The listing builds one solid part. Answer for the finished solid, in the listing's coordinates (mm). A direction names the side the tool comes from. Round coordinates to 2 decimals unless told otherwise and drop trailing zeros. Write each loop counter-clockwise with the first axis right and the second up, starting at its lowest first coordinate (ties: lowest second). Pieces come first, ordered by that corner, then holes.
(1) Each of these flat-tipped pins is pushed along its axis until it touches: pin 1 Ø2 at (x, y) = (-2.5, 9) entering from +Z; pin 2 Ø2 at (x, y) = (-8.5, 7) entering from +Z; pin 3 Ø2 at (y, z) = (11, 6) entering from -X. Where does it stop, or does it pass through?
(2) A cutting plane is placed at D-D, the plane z = -7. Give the vertices of the cut face in (x, y), and give its area (3 significant figures).
(3) Find the intervals of material crossed by probe 1 along Y at (x, z) = (0, 10); probe 2 along X at (y, z) = (9.75, 0) (3 decimals); probe 3 along X at (y, z) = (2.5, -4.75), in increasing order.
(4) The mould has two halves that part along X. Classify faces 3 (the face through (5.554, 7.148, -13.394)), 4 (the face through (8.12, 12.04, -9.35)): +X half, -X half, draft (parallel to the pull), parting line (faces both ways), or undercut.
(5) A cutting plane is placed at A-A, the plane x = 5.5. Give the vertices of the cut face in (y, z), and give its area (3 significant figures).
(6) For faces 1 (the face through (0, 1, 2.502)), 2 (the face through (4.8, 9.5, -4.6)), determine the directions among +Z, -Z, +X, -X, +Y, -Y from which every point of the face is accessible in a straight line to the end or side of a thin tool.
(7) A cutting plane is placed at B-B, the plane z = 0. Give the vertices of the cut face in (x, y) (3 decimals), and give its area (3 significant figures).
(8) A cutting plane is placed at C-C, the plane y = 11. Give the number of separate pieces and of enclosed holes in the cut face, and give its area (3 significant figures).
from build123d import *
from build123d.topology import SkipClean

# Parameters (mm, degrees)
CROQUIS1_R              = 14.5
SALIENTE_EXTRUIR1_DEPTH = 14.5
CORTAR_EXTRUIR1_DEPTH   = 26.11473671
CORTAR_EXTRUIR2_DEPTH   = 26.11473671
CORTAR_EXTRUIR3_DEPTH   = 5
MATRIZL1_COUNT          = 2
MATRIZL1_PITCH          = 12.728
MATRIZL1_COUNT_DIR2     = 2
MATRIZL1_PITCH_DIR2     = 12.728
CROQUIS6_R              = 2
CORTAR_EXTRUIR4_DEPTH   = 11.998295581
CORTAR_EXTRUIR5_DEPTH   = 1
CORTAR_EXTRUIR9_DEPTH   = 1.9


with BuildPart() as part:
    # Croquis1 → Saliente-Extruir1 (new body)
    with BuildSketch(Plane(origin=(0, 0, 0), x_dir=(1, 0, 0), z_dir=(0, 1, 0))):
        with Locations(Location((0, 0, 0), (0, 0, 90))):
            Circle(CROQUIS1_R)
    extrude(amount=SALIENTE_EXTRUIR1_DEPTH)

    # Croquis2 → Cortar-Extruir1 (cut, through all)
    with BuildSketch(Plane(origin=(0, 14.5, 0), x_dir=(1, 0, 0), z_dir=(0, 1, 0))):
        with BuildLine():
            Line((-1.61, -2.501704419), (1.61, -2.501704419))
            ThreePointArc((1.61, -2.501704419), (0, 2.975), (-1.61, -2.501704419))
        make_face()
    extrude(amount=-CORTAR_EXTRUIR1_DEPTH, mode=Mode.SUBTRACT)

    # Croquis3 → Cortar-Extruir2 (cut, through all)
    with BuildSketch(Plane(origin=(0, 14.5, 0), x_dir=(1, 0, 0), z_dir=(0, 1, 0))):
        with BuildLine():
            ThreePointArc((-4.364, 6.364), (-7.778213562, 7.778213562), (-6.364, 4.364))
            Line((-6.364, 4.364), (-6.364, 6.364))
            Line((-6.364, 6.364), (-4.364, 6.364))
        make_face()
        with BuildLine():
            Line((-6.364, 6.364), (-6.364, 4.364))
            ThreePointArc((-6.364, 4.364), (-4.949786438, 4.949786438), (-4.364, 6.364))
            Line((-4.364, 6.364), (-6.364, 6.364))
        make_face()
        with BuildLine():
            Line((-6.364, -4.364), (-6.364, -6.364))
            Line((-6.364, -6.364), (-4.364, -6.364))
            ThreePointArc((-4.364, -6.364), (-4.949786438, -4.949786438), (-6.364, -4.364))
        make_face()
        with BuildLine():
            Line((-4.364, -6.364), (-6.364, -6.364))
            Line((-6.364, -6.364), (-6.364, -4.364))
            ThreePointArc((-6.364, -4.364), (-7.778213562, -7.778213562), (-4.364, -6.364))
        make_face()
        with BuildLine():
            ThreePointArc((6.364, -4.364), (4.949786438, -4.949786438), (4.364, -6.364))
            Line((4.364, -6.364), (6.364, -6.364))
            Line((6.364, -6.364), (6.364, -4.364))
        make_face()
        with BuildLine():
            Line((6.364, -6.364), (4.364, -6.364))
            ThreePointArc((4.364, -6.364), (6.364, -8.364), (8.364, -6.364))
            ThreePointArc((8.364, -6.364), (7.778213562, -4.949786438), (6.364, -4.364))
            Line((6.364, -4.364), (6.364, -6.364))
        make_face()
        with BuildLine():
            ThreePointArc((4.364, 6.364), (4.949786438, 4.949786438), (6.364, 4.364))
            Line((6.364, 4.364), (6.364, 6.364))
            Line((6.364, 6.364), (4.364, 6.364))
        make_face()
        with BuildLine():
            Line((6.364, 6.364), (6.364, 4.364))
            ThreePointArc((6.364, 4.364), (7.778213562, 4.949786438), (8.364, 6.364))
            ThreePointArc((8.364, 6.364), (6.364, 8.364), (4.364, 6.364))
            Line((4.364, 6.364), (6.364, 6.364))
        make_face()
    extrude(amount=-CORTAR_EXTRUIR2_DEPTH, mode=Mode.SUBTRACT)

    # Croquis5 → Cortar-Extruir3 (cut)
    with BuildSketch(Plane(origin=(0, 14.5, 0), x_dir=(1, 0, 0), z_dir=(0, 1, 0))):
        Polygon((-6.364, 2.364), (-2.899898385, 4.364), (-2.899898385, 8.364), (-6.364, 10.364), (-9.828101615, 8.364), (-9.828101615, 4.364), align=None)
    cortar_extruir3 = extrude(amount=-CORTAR_EXTRUIR3_DEPTH, mode=Mode.SUBTRACT)

    # MatrizL1: Cortar-Extruir3 2 × 2
    with Locations(*[(i * MATRIZL1_PITCH, 0, j * MATRIZL1_PITCH_DIR2) for i in range(MATRIZL1_COUNT) for j in range(MATRIZL1_COUNT_DIR2) if (i, j) != (0, 0)]):
        add(cortar_extruir3, mode=Mode.SUBTRACT)

    # Croquis6 → Cortar-Extruir4 (cut)
    with BuildSketch(Plane.XY.offset(14.5)):
        with Locations((0, 10.5)):
            Circle(CROQUIS6_R)
        with Locations((0, 4.5)):
            Circle(CROQUIS6_R)
    extrude(amount=-CORTAR_EXTRUIR4_DEPTH, mode=Mode.SUBTRACT)

    # Croquis9 → Cortar-Extruir5 (cut)
    with SkipClean():  # the faces are left unmerged after this step: merging them gives an invalid solid
        with BuildSketch(Plane.XY.offset(2.501704419)):
            with BuildLine():
                Line((-1.61, 11.68654962), (-1.61, 9.31345038))
                ThreePointArc((-1.61, 9.31345038), (-2, 10.5), (-1.61, 11.68654962))
            make_face()
            with BuildLine():
                Line((1.61, 11.68654962), (1.61, 9.31345038))
                ThreePointArc((1.61, 9.31345038), (2, 10.5), (1.61, 11.68654962))
            make_face()
            with BuildLine():
                Line((-1.61, 5.68654962), (-1.61, 3.31345038))
                ThreePointArc((-1.61, 3.31345038), (-2, 4.5), (-1.61, 5.68654962))
            make_face()
            with BuildLine():
                Line((1.61, 5.68654962), (1.61, 3.31345038))
                ThreePointArc((1.61, 3.31345038), (2, 4.5), (1.61, 5.68654962))
            make_face()
        extrude(amount=-CORTAR_EXTRUIR5_DEPTH, mode=Mode.SUBTRACT)

    # Croquis11 → Cortar-Extruir9 (cut)
    with SkipClean():  # the faces are left unmerged after this step: merging them gives an invalid solid
        with BuildSketch(Plane(origin=(0, 14.5, 0), x_dir=(1, 0, 0), z_dir=(0, 1, 0))):
            with BuildLine():
                ThreePointArc((2.975, 0), (-1.424934209, 2.61154887), (-1.61, -2.501704419))
                Line((-1.61, -2.501704419), (1.61, -2.501704419))
                ThreePointArc((1.61, -2.501704419), (2.61154887, -1.424934209), (2.975, 0))
            make_face()
            with BuildLine():
                Line((1.61, -2.501704419), (-1.61, -2.501704419))
                ThreePointArc((-1.61, -2.501704419), (0, -2.975), (1.61, -2.501704419))
            make_face()
        extrude(amount=-CORTAR_EXTRUIR9_DEPTH, mode=Mode.SUBTRACT)


solid = part.part
Solutions:
1. pin 1: stops at z = 14.42
1. pin 2: stops at z = 12.41
1. pin 3: stops at x = -13.61
2. outline: (-12.7, 0) - (-8.26, 0) - (-8.26, 9.5) - (-9.83, 9.5) - (-9.83, 14.5) - (-12.7, 14.5) - close; (-4.47, 0) - (4.47, 0) - (4.47, 9.5) - (2.9, 9.5) - (2.9, 14.5) - (-2.9, 14.5) - (-2.9, 9.5) - (-4.47, 9.5) - close; (8.26, 0) - (12.7, 0) - (12.7, 14.5) - (9.83, 14.5) - (9.83, 9.5) - (8.26, 9.5) - close
2. area: 227 mm2
3. probe 1: y = 0 to 2.5, 6.5 to 8.5, 12.5 to 14.5
3. probe 2: x = -14.5 to -2.975, 2.975 to 14.5
3. probe 3: x = -13.7 to -7.55, -5.18 to 5.18, 7.55 to 13.7
4. face 3: parting line
4. face 4: undercut
5. outline: (0, -13.42) - (14.5, -13.42) - (14.5, -9.87) - (9.5, -9.87) - (9.5, -8.17) - (0, -8.17) - close; (0, -4.56) - (9.5, -4.56) - (9.5, -2.86) - (14.5, -2.86) - (14.5, 2.86) - (9.5, 2.86) - (9.5, 4.56) - (0, 4.56) - close; (0, 8.17) - (9.5, 8.17) - (9.5, 9.87) - (14.5, 9.87) - (14.5, 13.42) - (0, 13.42) - close
5. area: 251 mm2
6. face 1: +Y, -Y
6. face 2: +Y
7. outline: (-14.5, 0) - (-2.975, 0) - (-2.975, 14.5) - (-14.5, 14.5) - close; (2.975, 0) - (14.5, 0) - (14.5, 14.5) - (2.975, 14.5) - close
7. area: 334 mm2
8. separate pieces: 1
8. enclosed holes: 4
8. area: 421 mm2
